Source: three-view drawing plus pictorial views. Frame: mm from the lowest corner of the part. Give positions to 0.01 mm unless a question says otherwise; leave off trailing zeros. Order: outer loops, then holes, each group sorted by start corner. A loop starts at its lowest first (then second) coordinate and runs counter-clockwise, first axis right, second up. Notation, with made-up numbers: (-11, 10) - (1, 10) arc R18 ccw to (1, 36) - close; hole circle Ø3 at (31.5, -40). An arc over 180 degrees is marked (long way). Use one line per item in the form item = value.
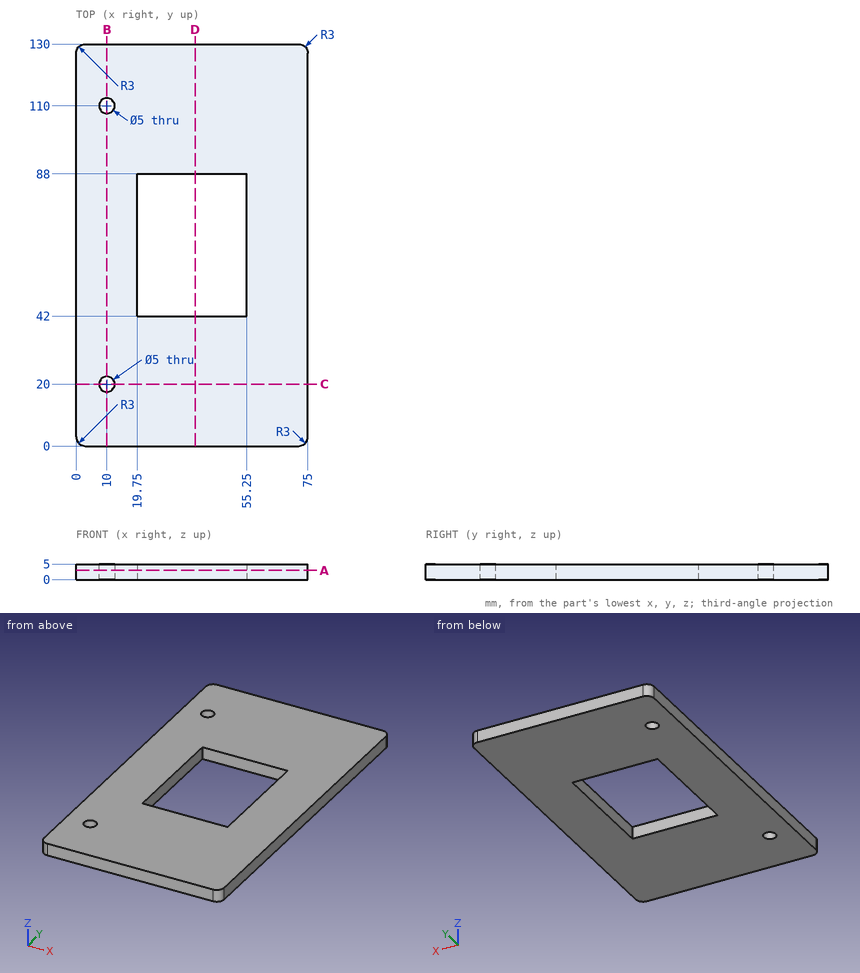
(1) Cut plane A-A on z = 2.95. Output: boundary loops of the cut face in (x, y), plus the area to 3 significant figures.
Computed values:
outline = (0, 3) arc R3 ccw to (3, 0) - (72, 0) arc R3 ccw to (75, 3) - (75, 127) arc R3 ccw to (72, 130) - (3, 130) arc R3 ccw to (0, 127) - close; hole circle Ø5 at (10, 20); hole circle Ø5 at (10, 110); hole (19.75, 42) - (55.25, 42) - (55.25, 88) - (19.75, 88) - close
area = 8,070 mm²
(2) Cut plane D-D on x = 38.5. Output: boundary loops of the cut face in (y, z), plus the area to 3 significant figures.
Computed values:
outline = (0, 0) - (42, 0) - (42, 5) - (0, 5) - close; (88, 0) - (130, 0) - (130, 5) - (88, 5) - close
area = 420 mm²
(3) Ray query, line 1 along Y through (x, z) = (10, 1.75); line 2 along Y through (x, z) = (41.5, 4.7); line 3 along X through (y, z) = (86.5, 3.45). Return the intervals inside material, ascending.
Computed values:
line_1 = 0 to 17.5, 22.5 to 107.5, 112.5 to 130
line_2 = 0 to 42, 88 to 130
line_3 = 0 to 19.75, 55.25 to 75
(4) Contact query for a flat-ended pin moving along its axis: pin 1 Ø3 at (x, y) = (10, 110) entering from +Z. Output: stop coordinate, or through.
Computed values:
pin_1 = through
(5) Cut plane B-B on x = 10. Output: boundary loops of the cut face in (y, z), plus the area to 3 significant figures.
Computed values:
outline = (0, 0) - (17.5, 0) - (17.5, 5) - (0, 5) - close; (22.5, 0) - (107.5, 0) - (107.5, 5) - (22.5, 5) - close; (112.5, 0) - (130, 0) - (130, 5) - (112.5, 5) - close
area = 600 mm²
(6) Cut plane C-C on y = 20. Output: boundary loops of the cut face in (x, z), plus the area to 3 significant figures.
Computed values:
outline = (0, 0) - (7.5, 0) - (7.5, 5) - (0, 5) - close; (12.5, 0) - (75, 0) - (75, 5) - (12.5, 5) - close
area = 350 mm²
